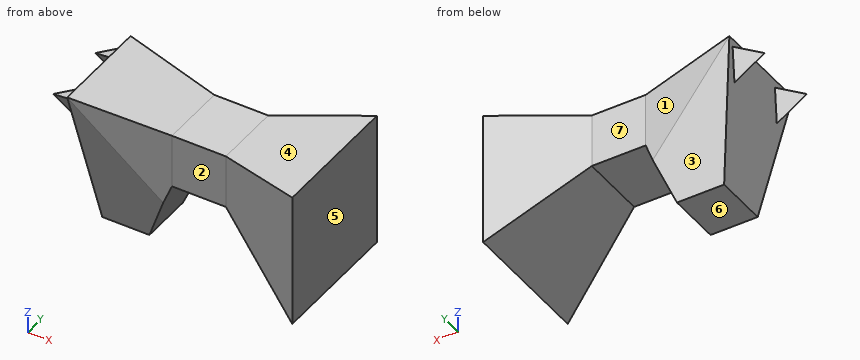
Autodesk Inventor part; units mm, degrees
ref_plane "Work Plane1" through (-40, 0, 0) normal (1, 0, 0) x (0, 0, -1)
ref_plane "Work Plane3" through (-43.9557, 2.5, -0.5934) normal (-0.9889364, 0, -0.1483405) x (-0.1483405, 0, 0.9889364)
ref_plane "Work Plane4" through (-37, 10, -42.4242) normal (0, 1, 0) x (1, 0, 0)
sketch "Sketch1" plane through (0, 0, 0) normal (0, 1, 0) x (-1, 0, 0)
  line L0 (0, 0) -> (40, 0)
  line L1 (0, 0) -> (0, -20)
  line L2 (0, 0) -> (0, -10)
  line L3 (37, -20) -> (40, 0)
  line L4 (37, -20) -> (30, -20)
  line L5 (26, -10) -> (30, -20)
  line L6 (26, -10) -> (18, -10)
  line L7 (0, -20) -> (5, -20)
  line L8 (5, -20) -> (18, -10)
  line L9 (18, 0) -> (18, -2)
  line L10 (18, -2) -> (5, 0)
  line L11 (18, -2) -> (26, -2)
  line L12 (26, -2) -> (40, 0)
  dimension "d1" = 40
  dimension "d2" = 20
  dimension "d7" = 10
  dimension "d8" = 37
  dimension "d9" = 7
  dimension "d10" = 26
  dimension "d11" = 8
  dimension "d12" = 5
  dimension "d33" = 2
extrude "Extrusion1" add sketch "Sketch1" along normal blind 20 contours L0 L10 L11 L12 L3 L4 L5 L6 L8 L7 L1
sketch "Sketch2" plane through (-40, 0, 0) normal (0, 0, 1) x (1, 0, 0)
  line L0 (3, 0) -> (3, 20)
  line L1 (10, 0) -> (10, 20)
  line L2 (14, 0) -> (14, 20)
  line L3 (22, 0) -> (22, 20)
  line L4 (35, 0) -> (35, 20)
  line L5 (40, 0) -> (40, 20)
  line L6 (0, 0) -> (0, 20)
  line L7 (0, 20) -> (40, 20)
  line L8 (35, 0) -> (40, 0)
  line L9 (40, 0) -> (40, 20)
  line L10 (35, 20) -> (40, 20)
  line L11 (40, 0) -> (40, 20)
  line L12 (40, 10) -> (0, 10)
  line L13 (22, 0) -> (22, 5)
  line L14 (35, 0) -> (22, 0)
  line L15 (22, 5) -> (35, 0)
  line L16 (22, 5) -> (14, 5)
  line L17 (10, 0) -> (10, 2.5)
  line L18 (10, 2.5) -> (14, 5)
  line L19 (10, 2.5) -> (3, 2.5)
  line L20 (22, 15) -> (35, 20)
  line L21 (22, 15) -> (14, 15)
  line L22 (10, 17.5) -> (14, 15)
  line L23 (10, 17.5) -> (3, 17.5)
  line L24 (3, 17.5) -> (0, 17.5)
  line L25 (3, 2.5) -> (0, 2.5)
  line L26 (14, 5) -> (0, 2.5)
  line L27 (14, 15) -> (0, 17.5)
  line L28 (35, 0) -> (35, 20)
  line L29 (0, 0) -> (14, 0)
  line L30 (0, 0) -> (40, 0)
  dimension "d15" = 5
  dimension "d16" = 2.5
extrude "Extrusion2" cut sketch "Sketch2" against normal blind 20 contours L29 L6 L25 L0 | L0 L19 L1 L29 | L25 L26 L0 | L0 L26 L1 L19 | L1 L18 L2 L29 | L1 L26 L18 | L2 L16 L3 L30 | L3 L15 L14 | L27 L24 L0 | L0 L23 L1 L27 | L6 L7 L0 L24 | L4 L12 L5 L8 | L0 L7 L1 L23 | L1 L22 L27 | L22 L1 L7 L2 | L2 L7 L3 L21 | L4 L7 L5 L12 | L3 L7 L20
ref_plane "Work Plane1" through (-40, 0, 0) normal (1, 0, 0) x (0, 0, -1)
sketch "Sketch4" plane through (-40, 0, 0) normal (1, 0, 0) x (0, 0, -1)
  line L0 (0, 17.5) -> (20, 16.9643)
  line L1 (20, 3.0357) -> (20, 16.9643)
  line L2 (20, 3.0357) -> (0, 2.5)
  line L3 (20, 3.0357) -> (20, 16.9643)
  line L4 (20, 3.0357) -> (20, 6.0357)
  line L5 (20, 16.9643) -> (20, 13.9643)
  line L6 (20, 4.2857) -> (20, 15.7143)
  line L7 (0, 2.5) -> (0, 17.5)
  line L8 (0, 2.5) -> (20, 6.0357)
  line L9 (0, 17.5) -> (20, 16.9643)
  line L10 (20, 13.9643) -> (0, 17.5)
  point P0 (0, 0)
  dimension "d24" = 3
  dimension "d25" = 3
extrude "Extrusion4" cut sketch "Sketch4" along normal blind 22 contours L0 L1 L10 | L8 L1 L2
sketch "Sketch5" plane through (-40, 2.5, 0) normal (-0.9889364, 0, -0.1483405) x (-0.1483405, 0, 0.9889364)
  line L0 (0, 0) -> (0, 15)
  line L1 (0, 14) -> (-1, 14)
  line L2 (-4.0546, 12.5) -> (-11.9661, 12.5)
  line L3 (-5.5, 12.5) -> (-1, 14)
  line L4 (0, 11) -> (-1, 11)
  line L5 (-1, 14) -> (-1, 11)
  line L6 (-5.5, 12.5) -> (-1, 11)
  point P0 (-5.9336, -2.5)
  point P1 (-4.8339, 12.5)
  dimension "d53" = 1
  dimension "d55" = 1
ref_plane "Work Plane3" through (-43.9557, 2.5, -0.5934) normal (-0.9889364, 0, -0.1483405) x (-0.1483405, 0, 0.9889364)
sketch "Sketch8" plane through (-43.9557, 2.5, -0.5934) normal (-0.9889364, 0, -0.1483405) x (-0.1483405, 0, 0.9889364)
  line L0 (-5.5, 12.5) -> (-1, 14)
  line L1 (-1, 14) -> (-1, 11)
  line L2 (-5.5, 12.5) -> (-1, 11)
  line L3 (-1, 12.5) -> (-2, 12.5)
  point P0 (-5.9336, -2.5)
  dimension "d56" = 1
loft "Loft3" add profiles "Sketch5" section 1 point at (-43.6591, 15, -2.5712) contours L6 L3 L5
ref_plane "Work Plane4" through (-37, 10, -42.4242) normal (0, 1, 0) x (1, 0, 0)
mirror "Mirror1" about plane through (-37, 10, -42.4242) normal (0, 1, 0) of "Loft3"
properties part number "horse"
Input: part model. Units: mm. Frame: model coordinates. Face numbers are marked on the shaded views. A direction names the side the tool comes from. Give positions to 0.01 mm unless a question says otherwise; leave off trailing zeros. Write each loop counter-clockwise with the first axis right and the second up, starting at its lowest first coordinate (ties: lowest second). Pieces come first, ordered by that corner, then holes. Notation, with made-up numbers: (86, 39.5) - (100, 39.5) arc R17 cw to (100, 55.5) - close; hole circle Ø7 at (88, -8). An arc over 180 degrees is marked (long way). Write item = value, one per line. Start each with the question number.
1. Ray query, L1, parallel to Z at x = -25, y = 5.5; L2, parallel to X at y = 5, z = -13.75 (1 decimal); L3, parallel to X at y = 6, z = -13.5 (3 decimals). Return the intervals inside material, ascending.
2. Section query D-D, the plane z = -3. Output: boundary loops of the cut face in (x, y), then the cut area to 3 significant figures.
3. Section query C-C, the plane y = 4. Output: boundary loops of the cut face in (x, z), then the cut area to 3 significant figures.
4. Access query for the marked faces 1, 2, 3 and 4. Directions: +Z, -Z, +X, -X, +Y, -Y. A direction counts if a zero-diameter tool reaches every point of the face in a straight line with its end or side. Return the directions, or none.
5. Mould query, pull axis X, two halves, no side actions, for the marked faces 5, 6 and 7. Classes: released by +X, released by -X, zero draft, split by the parting line, or undercut.
6. Section query A-A, the plane y = 11.25. Output: boundary loops of the cut face in (x, z), then the cut area to 3 significant figures.
7. Section query B-B, the plane z = -14.5. Output: boundary loops of the cut face in (x, y) (3 decimals).
8. First-contact query: pin 1 Ø6.5 at (x, y) = (-21.5, 12) entering from -Z; pin 2 Ø6 at (x, y) = (-14.5, 17.5) entering from +Z; pin 3 Ø3 at (x, z) = (-37.5, -2.5) entering from +Y. Flat tips, straight axial feed; report the tip coordinate or a pass-through.
Check sheet entries:
q1.L1 = -10 to -2
q1.L2 = -37.9 to -27.5, -13.1 to -5
q1.L3 = -37.975 to -27.4, -13.45 to -5
q2.outline = (-42.99, 5) - (-39.55, 4.18) - (-39.55, 3.03) - (-37.03, 3.03) - (-26, 5) - (-18, 5) - (-5, 0) - (-5, 20) - (-18, 15) - (-26, 15) - (-37.03, 16.97) - (-39.55, 16.97) - (-39.55, 15.82) - (-42.99, 15) - (-39.55, 14.18) - (-39.55, 5.82) - close
q2.area = 448 mm2
q3.outline = (-41.12, -1.52) - (-39.63, -2.47) - (-38.73, -8.48) - (-31.6, -8.48) - (-31.6, -1.2) - (-40, 0) - (-39.85, -0.99) - close; (-15.4, -12) - (-5, -20) - (-5, 0) - (-15.4, -1.6) - close
q3.area = 220 mm2
q4.face_1 = +Z, -Z, +Y
q4.face_2 = +Z, -Z, -Y
q4.face_3 = -Z, -X, +Y
q4.face_4 = +Z, +Y, -Y
q5.face_5 = released by +X
q5.face_6 = zero draft
q5.face_7 = undercut
q6.outline = (-40, 0) - (-37, -20) - (-30, -20) - (-26, -10) - (-18, -10) - (-5, -20) - (-5, 0) - (-18, -2) - (-26, -2) - close
q6.area = 462 mm2
q7.outline = (-37.825, 5.063) - (-27.8, 5.063) - (-27.8, 14.937) - (-37.825, 14.937) - close; (-12.15, 2.75) - (-5, 0) - (-5, 20) - (-12.15, 17.25) - close
q8.pin_1 = -10
q8.pin_2 = -1
q8.pin_3 = 17.24
